```python
from build123d import *

# Parameters (mm, degrees)
SKETCH2_R                = 14.463803576
BOSS_EXTRUDE1_DEPTH      = 2.5
BOSS_EXTRUDE1_TAPER      = 20
SKETCH4_W                = 8
SKETCH4_H                = 8
BOSS_EXTRUDE2_DEPTH      = 3
FILLET2_R                = 2
CIRPATTERN1_COUNT        = 4
FILLET2_OF_CIRPATTERN1_R = 2


with BuildPart() as part:
    # Sketch2 → Boss-Extrude1 (new body)
    with BuildSketch(Plane(origin=(0, 0, 0), x_dir=(1, 0, 0), z_dir=(0, 1, 0))):
        Circle(SKETCH2_R)
    extrude(amount=BOSS_EXTRUDE1_DEPTH, taper=BOSS_EXTRUDE1_TAPER)

    # Fillet1
    # an asymmetric fillet: 6, 4 mm, written as the material it takes off along each edge
    with BuildSketch(Plane(origin=(0, 2.5, 0), x_dir=(1, 0, 0), z_dir=(0, 0, -1))) as fillet1_piece_1:
        with BuildLine():
            Bezier((14.262848017, 1.94787914), (13.55387799, 0), (8.624692292, 0), weights=[1, 0.819152044, 1])
            Line((8.624692292, 0), (13.55387799, 0))
            Line((13.55387799, 0), (14.262848017, 1.94787914))
        make_face()
    revolve(axis=Axis((0, 2.5, 0), (0, -1, 0)), mode=Mode.SUBTRACT)

    # Sketch4 → Boss-Extrude2 (add)
    with BuildSketch(Plane(origin=(0, 0, 0), x_dir=(1, 0, 0), z_dir=(0, 1, 0))):
        with Locations((-12.616427752, -12.616427752)):
            Rectangle(SKETCH4_W, SKETCH4_H)
    boss_extrude2 = extrude(amount=BOSS_EXTRUDE2_DEPTH)

    # Fillet2
    fillet2_edges = [part.edges().sort_by_distance(p)[0] for p in [
        (-8.616427752, 1.5, 16.616427752),
        (-16.616427752, 1.5, 8.616427752),
        (-16.616427752, 1.5, 16.616427752),
    ]]
    fillet(fillet2_edges, radius=FILLET2_R)

    # CirPattern1: Boss-Extrude2 ×4 about axis, 1 skipped
    cirpattern1_axis = Axis((0, 0, 0), (0, 1, 0))
    add([boss_extrude2.rotate(cirpattern1_axis, i * 360 / CIRPATTERN1_COUNT) for i in range(1, CIRPATTERN1_COUNT) if i not in (1,)])

    # Fillet2 of CirPattern1
    fillet2_of_cirpattern1_edges = [part.edges().sort_by_distance(p)[0] for p in [
        (8.616427752, 1.5, -16.616427752),
        (16.616427752, 1.5, -8.616427752),
        (16.616427752, 1.5, -16.616427752),
        (-16.616427752, 1.5, -8.616427752),
        (-8.616427752, 1.5, -16.616427752),
        (-16.616427752, 1.5, -16.616427752),
    ]]
    fillet(fillet2_of_cirpattern1_edges, radius=FILLET2_OF_CIRPATTERN1_R)


solid = part.part
```
Here's how the part is built. I have some questions about the finished solid (model axes, mm). A direction names the side the tool comes from. Round coordinates to 2 decimals unless told otherwise and drop trailing zeros.
Q1. Will these pins go through, and if not, where does the flat tip stop? P1, Ø1, axis at x = -7, y = 0.5, coming from the +Z side; P2, Ø14, axis at x = 3.5, z = -3, coming from the +Y side.
Q2. If we mould it in two halves opening along Z, with no side actions, what happens to faces 3 (the flat face through (-13, 1, 16.616)), 4 (the flat face through (-12, 2, -8.616)), 5 (the flat face through (16.616, 1, -13)), 6 (the conical face through (-14.317, 0.403, -0.13))? For each: +Z half, -Z half, draft (parallel to the pull), parting line (faces both ways), or undercut.
Q3. Please list where these lines run through material, in increasing order: probe 1 along Z at (x, y) = (13.5, 2.85); probe 2 along Y at (x, z) = (2, -7.5); probe 3 along Z at (x, y) = (13, 0.55).
Q4. Which directions (+Z, -Z, +X, -X, +Y, -Y) give clear straight access to the entire face, cutting with the end or side of a thin tool? Please do faces 1 (the cylindrical face through (-16.05, 1.52, 9.22)), 2 (the flat face through (-13, 3, 13)).
Answer below:
1. P1: stops at z = 12.79
1. P2: stops at y = 2.5
2. face 3: +Z half
2. face 4: undercut
2. face 5: draft
2. face 6: undercut
3. probe 1: z = -16.62 to -8.62
3. probe 2: y = 0 to 2.5
3. probe 3: z = -16.62 to -8.62, -5.87 to 5.87
4. face 1: -X, +Y, -Y
4. face 2: +Z, -Z, +X, -X, +Y
